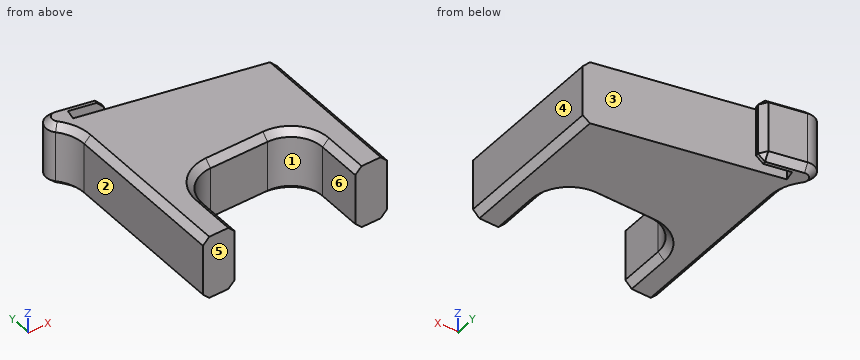
```python
from build123d import *

# Parameters (mm, degrees)
PAD_DEPTH            = 10
CHAMFER_SIZE         = 1
BODY_PLACEMENT_ANGLE = 270


with BuildPart() as part:
    # Sketch (on XZ_Plane of Origin) → Pad (new body)
    with BuildSketch(Plane.XZ):
        with BuildLine():
            Line((-1.5, 0), (-1.5, 25.451662))
            ThreePointArc((-1.5, 25.451662), (-1.901799, 27.610399), (-3.053383, 29.480011))
            ThreePointArc((-1.155354, 32.779089), (-3.304749, 31.820154), (-3.053383, 29.480011))
            Line((-1.155354, 32.779089), (5.202606, 31.427663))
            Line((5.202606, 31.427663), (4.890738, 29.960442))
            Line((4.890738, 29.960442), (0, 31))
            Line((0, 31), (-0.332659, 29.434964))
            Line((-0.332659, 29.434964), (27.5, 23.51895))
            Line((27.5, 23.51895), (27.5, 0))
            Line((27.5, 0), (22.5, 0))
            Line((22.5, 0), (22.5, 7))
            ThreePointArc((22.5, 7), (21.035534, 10.535534), (17.5, 12))
            Line((17.5, 12), (8.5, 12))
            ThreePointArc((8.5, 12), (4.964466, 10.535534), (3.5, 7))
            Line((3.5, 7), (3.5, 0))
            Line((3.5, 0), (-1.5, 0))
        make_face()
    extrude(amount=PAD_DEPTH)

    # Chamfer
    chamfer_edges = [part.edges().sort_by_distance(p)[0] for p in [
        (-1.5, -10, 12.725831),
        (3.5, -10, 3.5),
        (27.5, -10, 11.759475),
        (27.5, 0, 11.759475),
        (-1.5, 0, 12.725831),
        (22.5, 0, 3.5),
        (5.202606, -5, 31.427663),
        (5.046672, 0, 30.694052),
        (5.046672, -10, 30.694052),
    ]]
    chamfer(chamfer_edges, length=CHAMFER_SIZE)


with BuildPart() as part_1:
    # Body placement: moved
    add(part.part.rotate(Axis((0, 0, 0), (1, 0, 0)), BODY_PLACEMENT_ANGLE))


solid = part_1.part
```
Geometry check sheet. Reference: the model listing, model coordinates, mm. Face numbers are marked on the shaded views. A direction names the side the tool comes from. Coordinates: 2 decimals unless noted, no trailing zeros. Write each loop counter-clockwise with the first axis right and the second up, starting at its lowest first coordinate (ties: lowest second). Pieces come first, ordered by that corner, then holes. Notation, with made-up numbers: (-17, 9.5) -> (-9, 9.5) arc R22 cw to (-9, 39.5) -> close; hole circle Ø9 at (27, 46.25). An arc over 180 degrees is marked (long way). Use CSV: the item, a comma, the result in double quotes. Start each with the question number.
Item 1: Thickness scan on line 1 (X direction, y = 17.5, z = 6.5); line 2 (Y direction, x = 3, z = 7); line 3 (X direction, y = 11, z = 2.75). Record the ranges inside material, lowest first.
Item 2: Depth check by flat-ended pin: pin 1 Ø1.5 at (x, z) = (15.5, 5) entering from +Y; pin 2 Ø4 at (x, z) = (14, 3.5) entering from -Y; pin 3 Ø3.5 at (y, z) = (4.5, 5) entering from -X. Enter the tip coordinate at first touch or a pass-through.
Item 3: Cross-section at C-C, the plane x = 15.5. Record the cut outline in (y, z), plus the area to 3 significant figures.
Item 4: Cross-section at A-A, the plane z = 4.75. Record the cut outline in (x, y), plus the area to 3 significant figures.
Item 5: Mould release check, pull along X, two halves, no side actions. Record for the marked faces 4, 5 and 6: released by +X, released by -X, zero draft, split by the parting line, or undercut.
Item 6: Cross-section at B-B, the plane y = 15. Record the cut outline in (x, z), plus the area to 3 significant figures.
Item 7: Set-up check for the marked faces 1, 2 and 3: record each of +Z, -Z, +X, -X, +Y, -Y from which the full face is reachable in a straight line by a thin tool's end or side.
Item 8: Cross-section at D-D, the plane x = 9.5. Record the cut outline in (y, z), plus the area to 3 significant figures.
Answers:
1,line 1,"-1.5 to 27.5"
1,line 2,"0 to 28.73, 30.36 to 31.9"
1,line 3,"-1.5 to 5.5, 20.5 to 27.5"
2,pin 1,"y = 26.23"
2,pin 2,"y = 12"
2,pin 3,"x = -1.5"
3,outline,"(12, 1) -> (13, 0) -> (26.07, 0) -> (26.07, 10) -> (13, 10) -> (12, 9) -> close"
3,area,"140 mm^2"
4,outline,"(-3.05, 29.48) arc R6 cw to (-1.5, 25.45) -> (-1.5, 0) -> (3.5, 0) -> (3.5, 7) arc R5 cw to (8.5, 12) -> (17.5, 12) arc R5 cw to (22.5, 7) -> (22.5, 0) -> (27.5, 0) -> (27.5, 23.52) -> (-0.33, 29.43) -> (0, 31) -> (4.89, 29.96) -> (4.99, 30.45) -> (4.22, 31.64) -> (-1.16, 32.78) arc R2 ccw to start"
4,area,"574 mm^2"
5,face 4,"released by +X"
5,face 5,"zero draft"
5,face 6,"undercut"
6,outline,"(-1.5, 1) -> (-0.5, 0) -> (26.5, 0) -> (27.5, 1) -> (27.5, 9) -> (26.5, 10) -> (-0.5, 10) -> (-1.5, 9) -> close"
6,area,"288 mm^2"
7,face 1,"+Z, -Z, -Y"
7,face 2,"+Z, -Z, -X, -Y"
7,face 3,"+Z, -Z, +X"
8,outline,"(12, 1) -> (13, 0) -> (27.34, 0) -> (27.34, 10) -> (13, 10) -> (12, 9) -> close"
8,area,"152 mm^2"
